from build123d import *

# Parameters (mm, degrees)
EDIT_GLOBAL_VARIABLE_WITH_PCB_DIMENSIONS_W = 69.96
EDIT_GLOBAL_VARIABLE_WITH_PCB_DIMENSIONS_H = 102.98
BOSS_EXTRUDE1_DEPTH                        = 1.5
FILLET1_R                                  = 3
BOSS_EXTRUDE2_DEPTH                        = 91.1374
BOSS_EXTRUDE3_DEPTH                        = 91.1374
BOSS_EXTRUDE4_DEPTH                        = 58.1174
BOSS_EXTRUDE5_DEPTH                        = 58.1174
FILLET2_R                                  = 0.5
FILLET3_R                                  = 1


with BuildPart() as part:
    # EDIT GLOBAL VARIABLE WITH PCB DIMENSIONS → Boss-Extrude1 (new body)
    with BuildSketch(Plane(origin=(0, 0, 0), x_dir=(1, 0, 0), z_dir=(0, 1, 0))):
        Rectangle(EDIT_GLOBAL_VARIABLE_WITH_PCB_DIMENSIONS_W, EDIT_GLOBAL_VARIABLE_WITH_PCB_DIMENSIONS_H)
    extrude(amount=BOSS_EXTRUDE1_DEPTH)

    # Fillet1
    fillet1_edges = [part.edges().sort_by_distance(p)[0] for p in [
        (34.98, 0.75, 51.49),
        (-34.98, 0.75, 51.49),
        (-34.98, 0.75, -51.49),
        (34.98, 0.75, -51.49),
    ]]
    fillet(fillet1_edges, radius=FILLET1_R)

    # Sketch2 → Boss-Extrude2 (add)
    with BuildSketch(Plane.XY.offset(45.5687)):
        Polygon((33.18, 1.5), (29.058679656, 1.5), (32.119339828, 4.560660172), (33.18, 3.5), (32.18, 2.5), align=None)
    extrude(amount=-BOSS_EXTRUDE2_DEPTH)

    # Sketch3 → Boss-Extrude3 (add)
    with BuildSketch(Plane.XY.offset(45.5687)):
        Polygon((-33.18, 1.5), (-29.058679656, 1.5), (-32.119339828, 4.560660172), (-33.18, 3.5), (-32.18, 2.5), align=None)
    extrude(amount=-BOSS_EXTRUDE3_DEPTH)

    # Sketch4 → Boss-Extrude4 (add)
    with BuildSketch(Plane.ZY.offset(29.0587)):
        Polygon((-49.69, 1.5), (-45.568679656, 1.5), (-48.629339828, 4.560660172), (-49.69, 3.5), (-48.69, 2.5), align=None)
    extrude(amount=-BOSS_EXTRUDE4_DEPTH)

    # Sketch5 → Boss-Extrude5 (add)
    with BuildSketch(Plane.ZY.offset(29.0587)):
        Polygon((45.568679656, 1.5), (49.69, 1.5), (48.69, 2.5), (49.69, 3.5), (48.629339828, 4.560660172), align=None)
    extrude(amount=-BOSS_EXTRUDE5_DEPTH)

    # Fillet2
    fillet2_edges = [part.edges().sort_by_distance(p)[0] for p in [
        (33.18, 3.5, 0),
        (32.119339828, 4.560660172, 0),
        (-32.119339828, 4.560660172, 0),
        (-33.18, 3.5, 0),
        (0, 4.560660172, -48.629339828),
        (0, 3.5, -49.69),
        (0, 3.5, 49.69),
        (0, 4.560660172, 48.629339828),
    ]]
    fillet(fillet2_edges, radius=FILLET2_R)

    # Fillet3
    fillet3_edges = [part.edges().sort_by_distance(p)[0] for p in [
        (-34.98, 0, 0),
        (34.98, 0, 0),
        (0, 0, 51.49),
        (0, 0, -51.49),
        (-34.101320344, 0, 50.611320344),
        (34.101320344, 0, 50.611320344),
        (34.101320344, 0, -50.611320344),
        (-34.101320344, 0, -50.611320344),
    ]]
    fillet(fillet3_edges, radius=FILLET3_R)


solid = part.part
Could you check a few things on this model? Use its own coordinates, in mm. A direction names the side the tool comes from. Coordinates: 2 decimals unless noted, no trailing zeros. Order: outer loops, then holes, each group sorted by start corner. A loop starts at its lowest first (then second) coordinate and runs counter-clockwise, first axis right, second up. Notation, with made-up numbers: (50, 58) -> (98, 58) arc R8 ccw to (98, 64) -> close; hole circle Ø3 at (0, 71.5). An arc over 180 degrees is marked (long way). One line per item, written item: value. Start each with the question number.
1) Imagine slicing it at B-B on z = -5. List the corners of the cut face in (x, y) for me.
2) Which directions (+Z, -Z, +X, -X, +Y, -Y) give clear straight access to the entire face, cutting with the end or side of a thin tool? Please do faces 4 (the cylindrical face through (-34.12, 1.25, 50.59)), 5 (the flat face through (0, 1.5, -1)).
3) If I drill on L1, parallel to X at y = 0.8, z = 30; L2, parallel to Y at x = -13, z = 38; L3, parallel to X at y = 4.15, z = -8, over which ranges is the centre line in solid material (lowest first)? Write a range as [from, to].
4) Imagine slicing it at A-A on x = 2. List the corners of the cut face in (y, z) for me, plus the area to 3 significant figures.
5) We'd pull the mould along X, two halves only. Please class faces 1 (the flat face through (29.059, 3, 48)), 2 (the flat face through (-32, 3, -45.569)), 3 (the flat face through (30.39, 2.83, 0.64)): +X half, -X half, draft (parallel to the pull), parting line (faces both ways), or undercut.
6) I'm going to push flat-ended pins straight in: pin 1 (2 mm diameter, centred on x = 21.5, z = 2.5, fed in from +Y); pin 2 (1.4 mm diameter, centred on x = -30.5, y = 3, fed in from +Z); pin 3 (2.5 mm diameter, centred on y = 3.5, z = 47, fed in from +X). Where does each tip first touch, or does it pass through?
Answer list:
1. outline: (-34.98, 1) arc R1 ccw to (-33.98, 0) -> (33.98, 0) arc R1 ccw to (34.98, 1) -> (34.98, 1.5) -> (33.18, 1.5) -> (32.18, 2.5) -> (32.83, 3.15) arc R0.5 ccw to (32.83, 3.85) -> (32.47, 4.21) arc R0.5 ccw to (31.77, 4.21) -> (29.06, 1.5) -> (-29.06, 1.5) -> (-31.77, 4.21) arc R0.5 ccw to (-32.47, 4.21) -> (-32.83, 3.85) arc R0.5 ccw to (-32.83, 3.15) -> (-32.18, 2.5) -> (-33.18, 1.5) -> (-34.98, 1.5) -> close
2. face 4: +Z, -X, +Y, -Y
2. face 5: +Y
3. L1: x = [-34.96, 34.96]
3. L2: y = [0, 1.5]
3. L3: x = [-32.53, -31.71], [31.71, 32.53]
4. outline: (0, -50.49) arc R1 ccw to (1, -51.49) -> (1.5, -51.49) -> (1.5, -49.69) -> (2.5, -48.69) -> (3.15, -49.34) arc R0.5 ccw to (3.85, -49.34) -> (4.21, -48.98) arc R0.5 ccw to (4.21, -48.28) -> (1.5, -45.57) -> (1.5, 45.57) -> (4.21, 48.28) arc R0.5 ccw to (4.21, 48.98) -> (3.85, 49.34) arc R0.5 ccw to (3.15, 49.34) -> (2.5, 48.69) -> (1.5, 49.69) -> (1.5, 51.49) -> (1, 51.49) arc R1 ccw to (0, 50.49) -> close
4. area: 167 mm2
5. face 1: +X half
5. face 2: draft
5. face 3: undercut
6. pin 1: stops at y = 1.5
6. pin 2: stops at z = 45.57
6. pin 3: stops at x = 29.06
